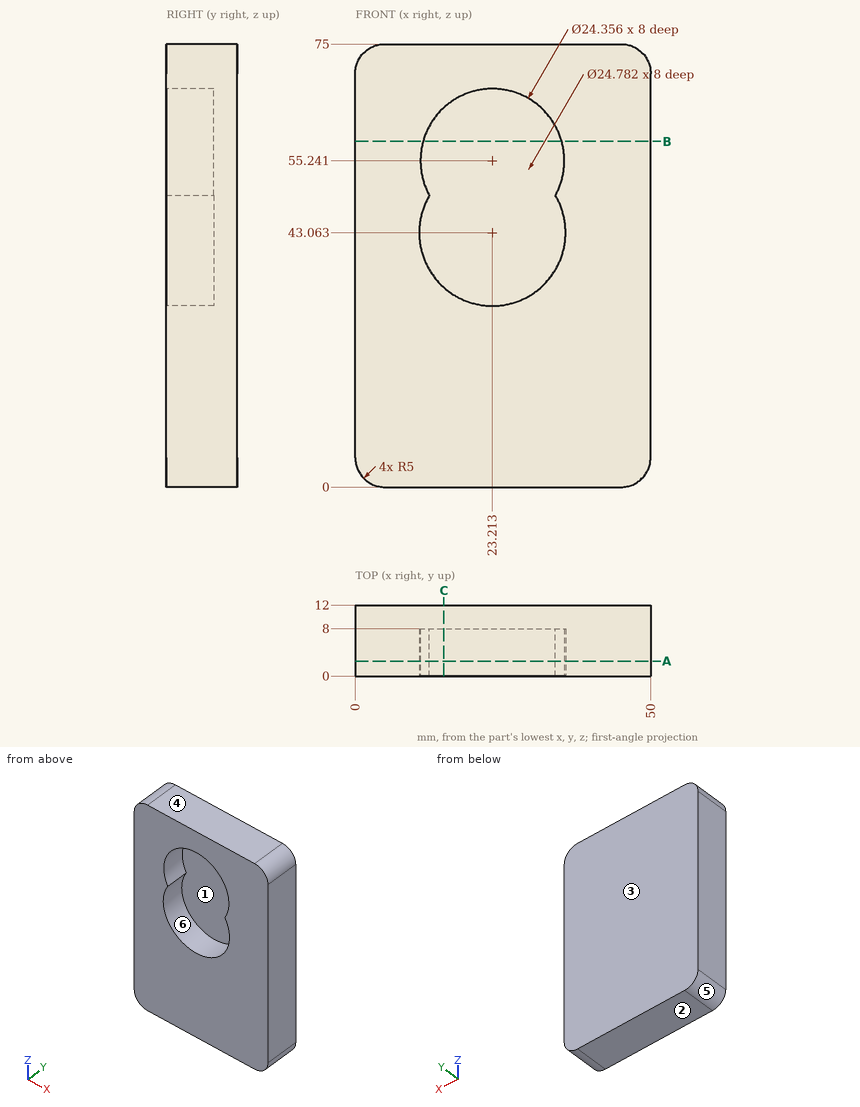
Source: three-view drawing plus pictorial views. Frame: mm from the lowest corner of the part. A direction names the side the tool comes from. Round coordinates to 2 decimals unless told otherwise and drop trailing zeros. Loops run counter-clockwise (first coordinate to the right, second up) from the corner with the lowest first, then second, coordinate; pieces in that order, holes last. Notation, with made-up numbers: M 7.25,-17 L 31.25,-17 A24 ccw 31.25,13 Z; hole C 1.5,50 d9. An arc over 180 degrees is marked long. Put each result on its own line as item: value. Start each with the question number.
(1) Section query A-A (y = 2.5). Return loops of the section in (x, z) (1 decimal).
(2) Draft query along Z for the marked faces 1, 2, 3 and 4. Return one class per face: +Z half, -Z half, draft (parallel to the pull), parting line (faces both ways), or undercut.
(3) Set-up query: the marked faces 5 and 6. Return all of +Z, -Z, +X, -X, +Y, -Y with unobstructed straight access to the full face (end or side cutting, diameter ignored); none if empty.
(4) Material intervals for line 1 along X through (y, z) = (3.75, 55.5); line 2 along Y through (x, z) = (26.5, 47); line 3 along X through (y, z) = (1.5, 58.5), sorted ascending. Write a range as [from, to].
(5) Section query B-B (z = 58.5). Return loops of the section in (x, y), then the cut area to 3 significant figures.
(6) Section query C-C (x = 15). Return loops of the section in (y, z) (1 decimal).
(7) Contact query for flat-ended pins moving along their axis: pin 1 Ø1 at (x, z) = (13, 39.5) entering from -Y; pin 2 Ø1.5 at (x, y) = (17, 3) entering from -Z. Output: stop coordinate, or through.
Findings below:
1. outline: M 0,5 A5 ccw 5,0 L 45,0 A5 ccw 50,5 L 50,70 A5 ccw 45,75 L 5,75 A5 ccw 0,70 Z; hole M 12.5,49.4 A12.4 ccw long 33.9,49.4 A12.2 ccw long Z
2. face 1: undercut
2. face 2: -Z half
2. face 3: draft
2. face 4: +Z half
3. face 5: -Z, -X, +Y, -Y
3. face 6: -Y
4. line 1: x = [0, 11.04], [35.39, 50]
4. line 2: y = [8, 12]
4. line 3: x = [0, 11.48], [34.95, 50]
5. outline: M 0,0 L 11.48,0 L 11.48,8 L 34.95,8 L 34.95,0 L 50,0 L 50,12 L 0,12 Z
5. area: 412 mm2
6. outline: M 0,0 L 12,0 L 12,75 L 0,75 L 0,64.2 L 8,64.2 L 8,33.8 L 0,33.8 Z
7. pin 1: stops at y = 8
7. pin 2: stops at z = 0
